Design review of the part built by this model. Coordinates are the model's own, in mm. A direction names the side the tool comes from. Coordinates: 2 decimals unless noted, no trailing zeros. Write each loop counter-clockwise with the first axis right and the second up, starting at its lowest first coordinate (ties: lowest second). Pieces come first, ordered by that corner, then holes. Notation, with made-up numbers: (6, 22.25) - (40, 22.25) arc R17 cw to (40, 47.25) - close; hole circle Ø1 at (-39, -21.5). An arc over 180 degrees is marked (long way). Answer as CSV lines item,"result". Start each with the question number.
Q1. We need section D-D (z = 22.5). Write out the cut boundary in (x, y).
Q2. We need section B-B (x = -34.5). Write out the cut boundary in (y, z).
Q3. Clearance check with flat-ended pins moving along their axes: pin 1 (0.6 mm diameter, centred on x = 23, z = 39, fed in from -Y); pin 2 (18 mm diameter, centred on x = 14, z = 19.5, fed in from -Y). State where each tip first meets the part, or that it passes through.
Q4. For line 1 along X through (y, z) = (-5.5, 7.5); line 2 along Z through (x, y) = (-3.5, 18.5); line 3 along Y through (x, z) = (22, 14.5), list the stretches that pass through material, from the lowest coordinate up. Write a range as [from, to].
Q5. Mouldability with a two-part tool opening along Z and no side actions: class faces 1 (the face through (-9, 13, 40)), 2 (the face through (-47.32, 2, 20)), 3 (the face through (-45.32, 1, 20)) as pulls with the +Z half, pulls with the -Z half, needs draft (parallel to the pull), parting line crosses it, or undercut.
Q6. Machinability: for faces 4 (the face through (52.68, 2, 20)), 5 (the face through (-27.32, -10, 39)), 6 (the face through (2, 23.84, 20)), which of the approach directions +Z, -Z, +X, -X, +Y, -Y give a long, thin tool a straight path to every point of the face, cutting with its end or side? Answer none if there is none.
Q7. We need section A-A (y = 17.5). Write out the cut boundary in (x, z), plus the area to 3 significant figures.
Q8. We need section C-C (y = -14.5). Write out the cut boundary in (x, z), plus the area to 3 significant figures.
from build123d import *

# Parameters (mm, degrees)
SKETCH1_W           = 100
SKETCH1_H           = 50
BOSS_EXTRUDE1_DEPTH = 40
SHELL1_T            = -2
SKETCH2_W           = 100
SKETCH2_H           = 40
CUT_EXTRUDE1_DEPTH  = 40
SKETCH3_W           = 96
SKETCH3_H           = 21
BOSS_EXTRUDE2_DEPTH = 38
SKETCH4_W           = 20
SKETCH4_H           = 48
BOSS_EXTRUDE3_DEPTH = 2
SHELL2_START        = -45.319513939
SHELL2_OUTLINE_W    = 21
SHELL2_OUTLINE_H    = 36
SHELL2_DEPTH        = 96


# Read off the part's stored shape, not the designer's step: Shell2
with BuildPart() as part:
    # Sketch1 → Boss-Extrude1 (new body)
    with BuildSketch(Plane.XY):
        with Locations((2.680486061, 0.839885633)):
            Rectangle(SKETCH1_W, SKETCH1_H)
    extrude(amount=BOSS_EXTRUDE1_DEPTH)

    # Shell1
    shell1_openings = [part.faces().sort_by_distance(p)[0] for p in [
        (2.680486061, 0.839885633, 40),
    ]]
    offset(amount=SHELL1_T, openings=shell1_openings, kind=Kind.INTERSECTION)

    # Sketch2 → Cut-Extrude1 (cut)
    with BuildSketch(Plane(origin=(0, -22.160114367, 0), x_dir=(1, 0, 0), z_dir=(0, 1, 0))):
        with Locations((2.680486061, -20)):
            Rectangle(SKETCH2_W, SKETCH2_H)
    extrude(amount=-CUT_EXTRUDE1_DEPTH, mode=Mode.SUBTRACT)

    # Sketch3 → Boss-Extrude2 (add)
    with BuildSketch(Plane.XY.offset(2)):
        with Locations((2.680486061, 13.339885633)):
            Rectangle(SKETCH3_W, SKETCH3_H)
    extrude(amount=BOSS_EXTRUDE2_DEPTH)

    # Sketch4 → Boss-Extrude3 (add)
    with BuildSketch(Plane.XY.offset(40)):
        with Locations((-37.319513939, 1.839885633)):
            Rectangle(SKETCH4_W, SKETCH4_H)
    extrude(amount=-BOSS_EXTRUDE3_DEPTH)

    # Shell2 outline → Shell2 (cut)
    with BuildSketch(Plane.YZ.offset(SHELL2_START)):
        with Locations((13.339885633, 20)):
            Rectangle(SHELL2_OUTLINE_W, SHELL2_OUTLINE_H)
    extrude(amount=SHELL2_DEPTH, mode=Mode.SUBTRACT)


solid = part.part
Results list:
1,outline,"(-47.32, -22.16) - (-45.32, -22.16) - (-45.32, 23.84) - (50.68, 23.84) - (50.68, -22.16) - (52.68, -22.16) - (52.68, 25.84) - (-47.32, 25.84) - close"
2,outline,"(-22.16, 0) - (25.84, 0) - (25.84, 40) - (-22.16, 40) - (-22.16, 38) - (23.84, 38) - (23.84, 2) - (-22.16, 2) - close"
3,pin 1,"stops at y = 2.84"
3,pin 2,"stops at y = 23.84"
4,line 1,"x = [-47.32, -45.32], [50.68, 52.68]"
4,line 2,"z = [0, 2], [38, 40]"
4,line 3,"y = [23.84, 25.84]"
5,face 1,"pulls with the +Z half"
5,face 2,"needs draft"
5,face 3,"undercut"
6,face 4,"+Z, -Z, +X, +Y, -Y"
6,face 5,"+Z, -Y"
6,face 6,"-Y"
7,outline,"(-47.32, 0) - (52.68, 0) - (52.68, 40) - (-47.32, 40) - close; hole (-45.32, 2) - (50.68, 2) - (50.68, 38) - (-45.32, 38) - close"
7,area,"544 mm2"
8,outline,"(-47.32, 0) - (52.68, 0) - (52.68, 40) - (50.68, 40) - (50.68, 2) - (-45.32, 2) - (-45.32, 38) - (-27.32, 38) - (-27.32, 40) - (-47.32, 40) - close"
8,area,"388 mm2"
